Design review of the part built by this model. Coordinates are the model's own, in mm. Face numbers are marked on the shaded views. Coordinates: 2 decimals unless noted, no trailing zeros. Loops run counter-clockwise (first coordinate to the right, second up) from the corner with the lowest first, then second, coordinate; pieces in that order, holes last.
Q1. For P1, Ø8, axis at x = 23, z = 39.5, coming from the +Y side; P2, Ø1, axis at x = -12.5, z = 104.5, coming from the -Y side; P3, Ø3, axis at x = -18, z = 50.5, coming from the +Y side, all flat-tipped, find the tip position at first contact; note any pin that passes through.
Q2. Add section A-A on y = 0. Give the boundary of the cut face in (x, z), and give its area (3 significant figures).
Q3. Draft analysis for pull direction Y (two halves, no side actions). For the marked faces 1 and 2, state which applies: released by +Y, released by -Y, zero draft, split by the parting line, or undercut.
Q4. Add section C-C on z = 138. Give the boundary of the cut face in (x, y), and give its area (3 significant figures).
Q5. Wall thickness on probe 1 along Y at (x, z) = (0, 31.5); probe 2 along Z at (x, y) = (-19, -13); probe 3 along X at (y, z) = (-22.5, 130): over which ranges is each line inside the solid? List them lowest first.
```python
from build123d import *

# Parameters (mm, degrees)
IZIM1_R                     = 67.5
IZIM1_R_2                   = 60
Y_KSEKLIK_EKSTR_ZYON1_DEPTH = 150
Y_KSEKLIK_EKSTR_ZYON2_START = 10
IZIM2_R                     = 67.5
Y_KSEKLIK_EKSTR_ZYON2_DEPTH = 10
RADYUS1_R                   = 5
RADYUS2_R                   = 5


with BuildPart() as part:
    # Çizim1 → Yükseklik-Ekstrüzyon1 (new body)
    with BuildSketch(Plane.XY):
        Circle(IZIM1_R)
        Circle(IZIM1_R_2, mode=Mode.SUBTRACT)
    extrude(amount=Y_KSEKLIK_EKSTR_ZYON1_DEPTH)

    # Çizim2 → Yükseklik-Ekstrüzyon2 (add)
    with BuildSketch(Plane(origin=(0, 0, 0), x_dir=(-1, 0, 0), z_dir=(0, 0, -1)).offset(Y_KSEKLIK_EKSTR_ZYON2_START)):
        Circle(IZIM2_R)
    extrude(amount=-Y_KSEKLIK_EKSTR_ZYON2_DEPTH)

    # Radyus1
    radyus1_edges = [part.edges().sort_by_distance(p)[0] for p in [
        (-67.5, 0, 150),
    ]]
    fillet(radyus1_edges, radius=RADYUS1_R)

    # Radyus2
    # the kernel refuses this fillet: 5 mm, written as the material it takes off along each edge
    with BuildSketch(Plane(origin=(0, 0, 150), x_dir=(1, 0, 0), z_dir=(0, -1, 0))) as radyus2_piece_1:
        with BuildLine():
            CenterArc((65, -4.330127019), RADYUS2_R, 120, 60)
            Line((60, -4.330127019), (59.9, -4.330127019))
            Line((59.9, -4.330127019), (59.9, 0))
            Line((59.9, 0), (60, 0.1))
            ThreePointArc((60, 0.1), (61.25, 0.1), (62.45, 0.08660254))
            Line((62.45, 0.08660254), (62.5, 0))
        make_face()
    revolve(axis=Axis((0, 0, 150), (0, 0, 1)), mode=Mode.SUBTRACT)


solid = part.part
```
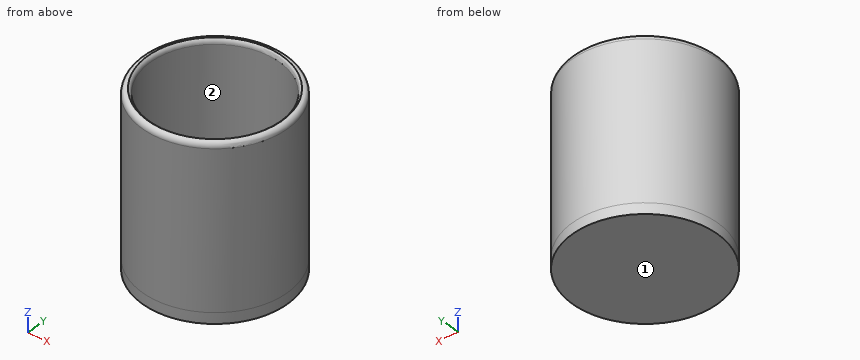
Entries:
1. P1: stops at y = 64.77
1. P2: stops at y = -66.42
1. P3: stops at y = 65.45
2. outline: (-67.5, -10) - (67.5, -10) - (67.5, 145) arc R5 ccw to (62.5, 150) arc R5 ccw to (60, 145.67) - (60, 0) - (-60, 0) - (-60, 145.67) arc R5 ccw to (-62.5, 150) arc R5 ccw to (-67.5, 145) - close
2. area: 3,580 mm2
3. face 1: zero draft
3. face 2: undercut
4. outline: circle Ø135 at (0, 0); hole circle Ø120 at (0, 0)
4. area: 3,000 mm2
5. probe 1: y = -67.5 to -60, 60 to 67.5
5. probe 2: z = -10 to 0
5. probe 3: x = -63.64 to -55.62, 55.62 to 63.64
